Model file for the job. Use its own axes, mm. A direction names the side the tool comes from. Coordinates: 2 decimals unless noted, no trailing zeros. Write each loop counter-clockwise with the first axis right and the second up, starting at its lowest first coordinate (ties: lowest second). Pieces come first, ordered by that corner, then holes. Notation, with made-up numbers: M 68,-26 L 79,-26 A25 ccw 79,-13 Z; hole C 3.25,89.5 d3. An arc over 180 degrees is marked long. Use CSV: the item, a comma, the result in double quotes. Start each with the question number.
from build123d import *

# Parameters (mm, degrees)
SKETCH1_R           = 1.7
SKETCH1_RX          = 25
SKETCH1_RY          = 17.67766953
BOSS_EXTRUDE1_DEPTH = 2
BOSS_EXTRUDE2_START = 2
SKETCH1_3_R         = 2.85
SKETCH1_3_R_2       = 26.3
BOSS_EXTRUDE2_DEPTH = 3
FILLET1_R           = 3


with BuildPart() as part:
    # Sketch1 → Boss-Extrude1 (new body)
    with BuildSketch(Plane(origin=(0, 50, 0), x_dir=(1, 0, 0), z_dir=(0, 1, 0))):
        with BuildLine():
            Line((-50, -35.67766953), (50, -35.67766953))
            ThreePointArc((50, -35.67766953), (57.071067812, -32.748737342), (60, -25.67766953))
            Line((60, -25.67766953), (60, 54.32233047))
            ThreePointArc((60, 54.32233047), (57.071067812, 61.393398282), (50, 64.32233047))
            Line((50, 64.32233047), (-50, 64.32233047))
            ThreePointArc((-50, 64.32233047), (-57.071067812, 61.393398282), (-60, 54.32233047))
            Line((-60, 54.32233047), (-60, -25.67766953))
            ThreePointArc((-60, -25.67766953), (-57.071067812, -32.748737342), (-50, -35.67766953))
        make_face()
        with Locations(Location((-50, -25.67766953, 0), (0, 0, 270))):
            Circle(SKETCH1_R, mode=Mode.SUBTRACT)
        with Locations(Location((50, -25.67766953, 0), (0, 0, 270))):
            Circle(SKETCH1_R, mode=Mode.SUBTRACT)
        with Locations(Location((50, 54.32233047, 0), (0, 0, 270))):
            Circle(SKETCH1_R, mode=Mode.SUBTRACT)
        with Locations(Location((-50, 54.32233047, 0), (0, 0, 270))):
            Circle(SKETCH1_R, mode=Mode.SUBTRACT)
        with Locations(Location((0, -0.777817459), (0, 0, -180))):
            Ellipse(SKETCH1_RX, SKETCH1_RY, mode=Mode.SUBTRACT)
    extrude(amount=BOSS_EXTRUDE1_DEPTH)

    # Sketch1<3> → Boss-Extrude2 (add)
    with BuildSketch(Plane(origin=(0, 50, 0), x_dir=(1, 0, 0), z_dir=(0, 1, 0)).offset(BOSS_EXTRUDE2_START)):
        with BuildLine():
            Line((-50, -35.67766953), (50, -35.67766953))
            ThreePointArc((50, -35.67766953), (57.071067812, -32.748737342), (60, -25.67766953))
            Line((60, -25.67766953), (60, 54.32233047))
            ThreePointArc((60, 54.32233047), (57.071067812, 61.393398282), (50, 64.32233047))
            Line((50, 64.32233047), (-50, 64.32233047))
            ThreePointArc((-50, 64.32233047), (-57.071067812, 61.393398282), (-60, 54.32233047))
            Line((-60, 54.32233047), (-60, -25.67766953))
            ThreePointArc((-60, -25.67766953), (-57.071067812, -32.748737342), (-50, -35.67766953))
        make_face()
        with Locations(Location((-50, 54.32233047, 0), (0, 0, 270))):
            Circle(SKETCH1_3_R, mode=Mode.SUBTRACT)
        with Locations(Location((-50, -25.67766953, 0), (0, 0, 270))):
            Circle(SKETCH1_3_R, mode=Mode.SUBTRACT)
        with Locations(Location((50, 54.32233047, 0), (0, 0, 270))):
            Circle(SKETCH1_3_R, mode=Mode.SUBTRACT)
        with Locations(Location((50, -25.67766953, 0), (0, 0, 270))):
            Circle(SKETCH1_3_R, mode=Mode.SUBTRACT)
        with Locations(Location((0, 0, 0), (0, 0, 270))):
            Circle(SKETCH1_3_R_2, mode=Mode.SUBTRACT)
    extrude(amount=BOSS_EXTRUDE2_DEPTH)

    # Fillet1
    fillet1_edges = [part.edges().sort_by_distance(p)[0] for p in [
        (57.071067812, 55, 32.748737342),
        (57.071067812, 55, -61.393398282),
        (-57.071067812, 55, -61.393398282),
        (-57.071067812, 55, 32.748737342),
        (60, 55, -14.32233047),
        (0, 55, -64.32233047),
        (-60, 55, -14.32233047),
        (0, 55, 35.67766953),
    ]]
    fillet(fillet1_edges, radius=FILLET1_R)


solid = part.part
1) Two-plate mould, pull along Z, no slides. Class faces 3 (the face through (-13, 55, -25)), 4 (the face through (-57.15, 50.99, 32.67)), 5 (the face through (47.218, 53.479, -54.94)): pulls with the +Z half, pulls with the -Z half, needs draft (parallel to the pull), parting line crosses it, or undercut.
2) Tool access for faces 1 (the face through (-51.034, 50.986, -55.671)), 2 (the face through (-52.782, 53.479, -54.94)): list every direction of +Z, -Z, +X, -X, +Y, -Y with a clear straight run to the whole face (end or side of a thin tool).
3) Wall check: L1, parallel to Z at x = -51, y = 50.3; L2, parallel to X at y = 54.5, z = -52.5; L3, parallel to Z at x = -11.5, y = 54.4. Give the ranges that are in metal, low to high. Write a range as [from, to].
4) Drop flat-ended pins along their axis: P1, Ø4, axis at x = 50, z = 25.68, coming from the +Y side; P2, Ø1, axis at x = -25.5, y = 53.5, coming from the +Z side. Give the stop position or say it passes through.
5) Band-saw the part on A-A on y = 53.65. List the corners of the cut face in (x, z), then the cut area to 3 significant figures.
Findings below:
1,face 3,"needs draft"
1,face 4,"pulls with the +Z half"
1,face 5,"undercut"
2,face 1,"+Y, -Y"
2,face 2,"+Y"
3,L1,"z = [-64.27, -55.7], [-52.95, 24.3], [27.05, 35.63]"
3,L2,"x = [-58.66, -52.19], [-47.81, 47.81], [52.19, 58.66]"
3,L3,"z = [-63.12, -23.65], [23.65, 34.48]"
4,P1,"stops at y = 52"
4,P2,"stops at z = 35.51"
5,outline,"M -59.51,-54.32 A9.51 ccw -50,-63.83 L 50,-63.83 A9.51 ccw 59.51,-54.32 L 59.51,25.68 A9.51 ccw 50,35.18 L -50,35.18 A9.51 ccw -59.51,25.68 Z; hole C -50,-54.32 d5.7; hole C -50,25.68 d5.7; hole C 0,0 d52.6; hole C 50,-54.32 d5.7; hole C 50,25.68 d5.7"
5,area,"9,430 mm2"
